Geometry: final body of the model. Coordinates: model frame, mm. A direction names the side the tool comes from. Round coordinates to 2 decimals unless told otherwise and drop trailing zeros. Use one line per item in the form item = value. Start each with the question number.
Item 1: Reachability of faces 1 (the flat face through (-7, 29, -44.45)), 2 (the flat face through (-7, 60.325, -73)), 3 (the flat face through (-7.299, 16.662, 43.504)), 4 (the flat face through (-7, 28, -47.625)), 5 (the flat face through (8, -3.175, 3)) from +Z, -Z, +X, -X, +Y, -Y: full face, straight path, thin tool, end or side. Return the list, or none.
Item 2: Pull-direction query (Z, two-part tool) for faces 6 (the flat face through (8, 0, 3)), 7 (the flat face through (-521.335, 35, -47)), 8 (the flat face through (-7.299, 17.921, 46.444)); classes: pulls with the +Z half, pulls with the -Z half, needs draft (parallel to the pull), parting line crosses it, or undercut.
Item 3: Ray query, probe 1 along X at (y, z) = (-1.55, 25.4); probe 2 along X at (y, z) = (12, -46) (3 decimals); probe 3 along Z at (x, y) = (584.2, -1.15). Return the intervals inside material, ascending.
Item 4: Pin query (flat end, axial travel): pin 1 Ø2 at (x, y) = (459, 34.5) entering from -Z (3 decimals); pin 2 Ø8 at (x, z) = (584.2, -25.4) entering from +Y; pin 3 Ø8 at (x, z) = (546.1, -25.4) entering from -Y (3 decimals); pin 4 Ø4 at (x, z) = (-0.635, -85.725) entering from -Y. Return the tip coordinate at first contact, or that it passes through.
from build123d import *

# Parameters (mm, degrees)
BASE_FLANGE1_DEPTH               = 3.175
EDGE_FLANGE1_START               = -521.335
EDGE_FLANGE1_DEPTH               = 1042.67
EDGE_FLANGE1_START_2             = -521.760369343
EDGE_FLANGE1_2_DEPTH             = 0.425369343
EDGE_FLANGE1_START_3             = 521.335
EDGE_FLANGE1_3_DEPTH             = 0.425369343
EDGE_FLANGE1_4_DEPTH             = 1042.67
EDGE_FLANGE2_DEPTH               = 1042.67
EDGE_FLANGE3_STRIP_W             = 19.05
EDGE_FLANGE3_STRIP_H             = 3.175
EDGE_FLANGE3_STRIP_CUT_DEPTH     = 1042.67
EDGE_FLANGE3_DEPTH               = 1042.67
FILLET1_R                        = 3.175
F_17_64_0_26563_DIAMETER_HOLE1_D = 6.747002
F_1_4_0_25_DIAMETER_HOLE1_D      = 6.35
F_1_4_0_25_DIAMETER_HOLE2_D      = 6.35
F_1_4_0_25_DIAMETER_HOLE2_DEPTH  = 3.175


# Read off the part's stored shape, not the designer's step: Edge-Flange1
# Sheet-metal steps are written as plain solids
with BuildPart() as part:
    # Sketch1 → Base-Flange1 (new body)
    with BuildSketch(Plane(origin=(0, 0, 0), x_dir=(1, 0, 0), z_dir=(0, 1, 0))):
        with BuildLine():
            Line((-521.335, 41.275), (-521.335, 47.625))
            Line((-521.335, 47.625), (521.335, 47.625))
            Line((521.335, 47.625), (521.335, 41.275))
            ThreePointArc((521.335, 41.275), (522.26493597, 39.02993597), (524.51, 38.1))
            Line((524.51, 38.1), (594.36, 38.1))
            Line((594.36, 38.1), (594.36, -38.1))
            Line((594.36, -38.1), (524.51, -38.1))
            ThreePointArc((524.51, -38.1), (522.26493597, -39.02993597), (521.335, -41.275))
            Line((521.335, -41.275), (521.335, -47.625))
            Line((521.335, -47.625), (-521.335, -47.625))
            Line((-521.335, -47.625), (-521.335, -41.275))
            ThreePointArc((-521.335, -41.275), (-522.26493597, -39.02993597), (-524.51, -38.1))
            Line((-524.51, -38.1), (-594.36, -38.1))
            Line((-594.36, -38.1), (-594.36, 38.1))
            Line((-594.36, 38.1), (-524.51, 38.1))
            ThreePointArc((-524.51, 38.1), (-522.26493597, 39.02993597), (-521.335, 41.275))
        make_face()
    extrude(amount=-BASE_FLANGE1_DEPTH)

    # Edge-Flange1 outline → Edge-Flange1 (cut)
    with BuildSketch(Plane.YZ.offset(EDGE_FLANGE1_START)):
        with BuildLine():
            ThreePointArc((0, -46.774261315), (-2.324261314, -44.450000001), (-3.175, -41.275))
            Line((-3.175, -41.275), (-3.175, -47.625))
            Line((-3.175, -47.625), (0, -47.625))
            Line((0, -47.625), (0, -46.774261315))
        make_face()
    extrude(amount=EDGE_FLANGE1_DEPTH, mode=Mode.SUBTRACT)

    # Edge-Flange1 2 outline → Edge-Flange1 2 (cut)
    with BuildSketch(Plane.YZ.offset(EDGE_FLANGE1_START_2)):
        with BuildLine():
            Line((0, -39.6875), (-3.175, -39.6875))
            Line((-3.175, -39.6875), (-3.175, -41.275))
            ThreePointArc((-3.175, -41.275), (-2.324261314, -44.450000001), (0, -46.774261315))
            Line((0, -46.774261315), (0, -39.6875))
        make_face()
    extrude(amount=EDGE_FLANGE1_2_DEPTH, mode=Mode.SUBTRACT)

    # Edge-Flange1 3 outline → Edge-Flange1 3 (cut)
    with BuildSketch(Plane.YZ.offset(EDGE_FLANGE1_START_3)):
        with BuildLine():
            Line((0, -39.6875), (-3.175, -39.6875))
            Line((-3.175, -39.6875), (-3.175, -41.275))
            ThreePointArc((-3.175, -41.275), (-2.324261314, -44.450000001), (0, -46.774261315))
            Line((0, -46.774261315), (0, -39.6875))
        make_face()
    extrude(amount=EDGE_FLANGE1_3_DEPTH, mode=Mode.SUBTRACT)

    # Edge-Flange1 4 outline → Edge-Flange1 4 (add)
    with BuildSketch(Plane.YZ.offset(EDGE_FLANGE1_START)):
        with BuildLine():
            ThreePointArc((3.175, -44.45), (0.92993597, -43.52006403), (0, -41.275))
            Line((0, -41.275), (0, -46.774261315))
            ThreePointArc((0, -46.774261315), (1.531499064, -47.408628997), (3.175, -47.625))
            Line((3.175, -47.625), (60.325, -47.625))
            Line((60.325, -47.625), (60.325, -44.45))
            Line((60.325, -44.45), (3.175, -44.45))
        make_face()
    extrude(amount=EDGE_FLANGE1_4_DEPTH)

    # Edge-Flange2 section (across the edge) → Edge-Flange2 (add)
    with BuildSketch(Plane(origin=(-521.335, 0, 53.124261314), x_dir=(0, -0.499999999999998, -0.8660254037844398), z_dir=(1, 0, 0))):
        with BuildLine():
            Line((-3.175, 5.499261314), (-3.175, 32.600738686))
            Line((-3.175, 32.600738686), (0, 32.600738686))
            Line((0, 32.600738686), (0, 5.499261314))
            ThreePointArc((0, 5.499261314), (1.5875, 2.749630657), (4.7625, 2.749630657))
            Line((4.7625, 2.749630657), (6.35, 0))
            ThreePointArc((6.35, 0), (0, 0), (-3.175, 5.499261314))
        make_face()
    extrude(amount=EDGE_FLANGE2_DEPTH)

    # Edge-Flange3 strip (across the edge) → Edge-Flange3 strip cut (cut)
    with BuildSketch(Plane(origin=(-521.335, 60.325, -47.625), x_dir=(0, -1, 0), z_dir=(1, 0, 0))):
        with Locations((-3.175, -1.5875)):
            Rectangle(EDGE_FLANGE3_STRIP_W, EDGE_FLANGE3_STRIP_H)
    extrude(amount=EDGE_FLANGE3_STRIP_CUT_DEPTH, mode=Mode.SUBTRACT)

    # Edge-Flange3 section (across the edge) → Edge-Flange3 (add)
    with BuildSketch(Plane(origin=(-521.335, 60.325, -47.625), x_dir=(0, -1, 0), z_dir=(1, 0, 0))):
        with BuildLine():
            Line((0, 3.175), (0, 47.625))
            Line((0, 47.625), (3.175, 47.625))
            Line((3.175, 47.625), (3.175, 3.175))
            ThreePointArc((3.175, 3.175), (4.10493597, 0.92993597), (6.35, 0))
            Line((6.35, 0), (6.35, -3.175))
            ThreePointArc((6.35, -3.175), (1.859871939, -1.315128061), (0, 3.175))
        make_face()
    extrude(amount=EDGE_FLANGE3_DEPTH)

    # Fillet1
    fillet1_edges = [part.edges().sort_by_distance(p)[0] for p in [
        (-521.335, 29.026817884, 38.1987073),
        (521.335, 29.026817884, 38.1987073),
        (-521.335, 58.7375, -95.25),
        (521.335, 58.7375, -95.25),
        (594.36, -1.5875, -38.1),
        (594.36, -1.5875, 38.1),
        (-594.36, -1.5875, 38.1),
        (-594.36, -1.5875, -38.1),
    ]]
    fillet(fillet1_edges, radius=FILLET1_R)

    # 17/64 (0.26563) Diameter Hole1 (through all)
    with Locations(Plane(origin=(0, -3.175, 0), x_dir=(-1, 0, 0), z_dir=(0, -1, 0))):
        with Locations((-546.1, 25.4), (-584.2, 25.4), (-584.2, -25.4), (-546.1, -25.4), (546.1, 25.4), (584.2, 25.4), (584.2, -25.4), (546.1, -25.4)):
            Hole(F_17_64_0_26563_DIAMETER_HOLE1_D / 2)

    # 1/4 (0.25) Diameter Hole1 (through all)
    with Locations(Plane(origin=(0, 57.15, 0), x_dir=(-1, 0, 0), z_dir=(0, -1, 0))):
        with Locations((-507.365, 85.725), (-507.365, 60.325), (-253.365, 85.725), (-253.365, 60.325), (0.635, 85.725), (0.635, 60.325), (254.635, 85.725), (254.635, 60.325), (508.635, 85.725), (508.635, 60.325)):
            Hole(F_1_4_0_25_DIAMETER_HOLE1_D / 2)

    # 1/4 (0.25) Diameter Hole2
    with Locations(Plane(origin=(0, 0, -47.625), x_dir=(-1, 0, 0), z_dir=(0, 0, -1))):
        with Locations((508.635, 44.45), (508.635, 12.7), (254.635, 44.45), (254.635, 12.7), (0, 44.45), (0.635, 12.7), (-253.365, 44.45), (-253.365, 12.7), (-507.365, 44.45), (-507.365, 12.7)):
            Hole(F_1_4_0_25_DIAMETER_HOLE2_D / 2, depth=F_1_4_0_25_DIAMETER_HOLE2_DEPTH)


solid = part.part
Working result:
q1.face_1 = +X, -X, +Y
q1.face_2 = +Z, -Z, +X, -X, +Y
q1.face_3 = +X, -X
q1.face_4 = -Z, +X, -X, -Y
q1.face_5 = +Z, -Z, +X, -X, -Y
q2.face_6 = undercut
q2.face_7 = needs draft
q2.face_8 = pulls with the +Z half
q3.probe_1 = -594.36 to -587.57, -580.83 to -549.47, -542.73 to 542.73, 549.47 to 580.83, 587.57 to 594.36
q3.probe_2 = -521.335 to -511.732, -505.538 to -257.732, -251.538 to -3.732, 2.462 to 250.268, 256.462 to 504.268, 510.462 to 521.335
q3.probe_3 = -38.1 to -28.77, -22.03 to 22.03, 28.77 to 38.1
q4.pin_1 = -47.625
q4.pin_2 = 0
q4.pin_3 = -3.175
q4.pin_4 = through
